```python
from build123d import *

# Parameters (mm, degrees)
SKETCH2_W          = 20
SKETCH2_H          = 15
CUT_EXTRUDE1_DEPTH = 200
SKETCH3_R          = 100
CUT_EXTRUDE2_DEPTH = 200


with BuildPart() as part:
    # Sketch1 → Revolve2 (revolve)
    with BuildSketch(Plane.XY, mode=Mode.PRIVATE) as revolve2_sk:
        with BuildLine():
            Line((-75, 25), (75, 25))
            Line((75, 25), (100, 25))
            Line((100, 25), (100, 75))
            Line((100, 75), (75, 75))
            Line((75, 75), (75, 462.5))
            Line((75, 462.5), (100, 462.5))
            Line((100, 462.5), (100, 512.5))
            Line((100, 512.5), (75, 512.5))
            ThreePointArc((75, 512.5), (0, 437.5), (-75, 512.5))
            Line((-75, 512.5), (-100, 512.5))
            Line((-100, 512.5), (-100, 462.5))
            Line((-100, 462.5), (-75, 462.5))
            Line((-75, 462.5), (-75, 75))
            Line((-75, 75), (-100, 75))
            Line((-100, 75), (-100, 25))
            Line((-100, 25), (-75, 25))
        make_face()
    revolve(revolve2_sk.sketch.rotate(Axis((-60.76079066, 0, 0), (1, 0, 0)), 90), axis=Axis((-60.76079066, 0, 0), (1, 0, 0)))

    # Sketch2 → Cut-Extrude1 (cut)
    with BuildSketch(Plane(origin=(100, 0, 0), x_dir=(0, 0, -1), z_dir=(1, 0, 0))):
        with Locations((0, 30.412878475)):
            Rectangle(SKETCH2_W, SKETCH2_H)
    extrude(amount=-CUT_EXTRUDE1_DEPTH, mode=Mode.SUBTRACT)

    # Sketch3 → Cut-Extrude2 (cut)
    with BuildSketch(Plane(origin=(75, 0, 0), x_dir=(0, 0, -1), z_dir=(1, 0, 0))):
        with Locations((0, -268.75)):
            Circle(SKETCH3_R)
        with Locations((-255.596438754, -83.048317238)):
            Circle(SKETCH3_R)
        with Locations((-157.967286554, 217.423317238)):
            Circle(SKETCH3_R)
        with Locations((157.967286554, 217.423317238)):
            Circle(SKETCH3_R)
        with Locations((255.596438754, -83.048317238)):
            Circle(SKETCH3_R)
    extrude(amount=-CUT_EXTRUDE2_DEPTH, mode=Mode.SUBTRACT)


solid = part.part
```
The model under review builds one solid part; all positions refer to its coordinate system, in mm. A direction names the side the tool comes from. Round coordinates to 2 decimals unless told otherwise and drop trailing zeros. Write each loop counter-clockwise with the first axis right and the second up, starting at its lowest first coordinate (ties: lowest second). Pieces come first, ordered by that corner, then holes.
(1) We need section B-B on z = -227.5. Give the number of separate pieces and of enclosed holes in the cut face, and give its area (3 significant figures).
(2) Mouldability with a two-part tool opening along Y and no side actions: class faces 4 (the cylindrical face through (1.05, -184.43, -53.76)), 5 (the cylindrical face through (87.325, -153.941, 488.834)), 6 (the cylindrical face through (1.05, 247.461, 62.585)), 7 (the flat face through (100, -458, 78)) as +Y half, -Y half, draft (parallel to the pull), parting line (faces both ways), or undercut.
(3) We need section A-A on x = 2. Give the boundary of the cut face in (y, z), and give its area (3 significant figures).
(4) Machinability: for faces 1 (the cylindrical face through (-87.325, -138.922, 441.143)), 2 (the cylindrical face through (1.05, -53.01, -350.98)), 3 (the cylindrical face through (87.675, -138.922, 441.143)), which of the approach directions +Z, -Z, +X, -X, +Y, -Y give a long, thin tool a straight path to every point of the face, cutting with its end or side? Answer none if there is none.
(5) Wall thickness on L1, parallel to Z at x = -37, y = 8.5; L2, parallel to Z at x = -18, y = 250.5; L3, parallel to Z at x = -50, y = 296.5: over which ranges is each line inside the solid? List them lowest first.
(6) Insertion check: pin 1 (2 mm diameter, centred on y = -194.5, z = 178, fed in from -X); pin 2 (7.5 mm diameter, centred on x = 30, y = 28.5, fed in from -Z); pin 3 (2 mm diameter, centred on x = 52.5, y = -152.5, fed in from -Z). Each pin has a flat end and moves straight along its axis. Give the tip position at first contact, or say it passes through.
Findings below:
1. separate pieces: 3
1. enclosed holes: 0
1. area: 73,000 mm2
2. face 4: undercut
2. face 5: parting line
2. face 6: undercut
2. face 7: draft
3. outline: circle Ø875.05 at (0, 0); hole circle Ø200 at (-268.75, 0); hole circle Ø200 at (-83.05, -255.6); hole circle Ø200 at (-83.05, 255.6); hole (22.91, -10) - (37.91, -10) - (37.91, 10) - (22.91, 10) arc R25 ccw (long way) to start; hole circle Ø200 at (217.42, -157.97); hole circle Ø200 at (217.42, 157.97)
3. area: 442,000 mm2
4. face 1: -X
4. face 2: +X, -X
4. face 3: +X
5. L1: z = -447.18 to -295.83, -215.36 to -23.51, 23.51 to 215.36, 295.83 to 447.18
5. L2: z = -361.36 to -252.34, -63.6 to 63.6, 252.34 to 361.36
5. L3: z = -347.23 to -219.18, -96.76 to 96.76, 219.18 to 347.23
6. pin 1: stops at x = -75
6. pin 2: stops at z = -444.63
6. pin 3: stops at z = -433.98
